Read the model definition and answer for the solid it produces. Units are mm, in the model's axes. Round coordinates to 2 decimals unless told otherwise and drop trailing zeros. Order: outer loops, then holes, each group sorted by start corner. A loop starts at its lowest first (then second) coordinate and runs counter-clockwise, first axis right, second up. Notation, with made-up numbers: (14.5, 49) - (38.5, 49) arc R34 cw to (38.5, 86) - close; hole circle Ø4 at (2.5, -34). An arc over 180 degrees is marked (long way). Put each result on its own line as item: value. Start each with the question number.
Q1. Section A-A on z = 12.5 is taken. Give the vertices of the cut face in (x, y), then the cut area to 3 significant figures.
Q2. Find the intervals of material crossed by line 1 along Y through (x, z) = (-0.25, 10); line 2 along Z through (x, y) = (0, 11.5); line 3 along X through (y, z) = (-4.25, 7.5), in increasing order. Write a range as from..to.
Q3. Section C-C on y = -2 is taken. Give the vertices of the cut face in (x, z), then the cut area to 3 significant figures.
Q4. This flat-tipped pin is pushed along its axis until it touches: pin 1 Ø0.6 at (x, y) = (-4, 7.5) entering from +Z. Where does it stop, or does it pass through?
Q5. Section B-B on y = 10.5 is taken. Give the vertices of the cut face in (x, z).
Q6. Section D-D on z = 3.5 is taken. Give the vertices of the cut face in (x, y), then the cut area to 3 significant figures.
from build123d import *

# Parameters (mm, degrees)
SKETCH027_W     = 15
SKETCH027_H     = 30
PAD008_DEPTH    = 15
SKETCH028_R     = 2
POCKET019_DEPTH = 29
SKETCH029_W     = 0.5
SKETCH029_H     = 17
POCKET020_DEPTH = 10
SKETCH030_W     = 7.783355
SKETCH030_H     = 0.5
POCKET021_DEPTH = 12
FILLET010_R     = 1.5
CHAMFER005_SIZE = 1


with BuildPart() as part:
    # Sketch027 → Pad008 (new body)
    with BuildSketch(Plane.XY):
        Rectangle(SKETCH027_W, SKETCH027_H)
    extrude(amount=PAD008_DEPTH)

    # Sketch028 (on Face3 of Pad008) → Pocket019 (cut)
    with BuildSketch(Plane.XZ.offset(15)):
        with Locations((0, 7.5)):
            Circle(SKETCH028_R)
    extrude(amount=-POCKET019_DEPTH, mode=Mode.SUBTRACT)

    # Sketch029 (on Face5 of Pocket019) → Pocket020 (cut)
    with BuildSketch(Plane.XY.offset(15)):
        with Locations((0.25, 0)):
            Rectangle(SKETCH029_W, SKETCH029_H)
    extrude(amount=-POCKET020_DEPTH, mode=Mode.SUBTRACT)

    # Sketch030 (on Face5 of Pocket020) → Pocket021 (cut)
    with BuildSketch(Plane.XY.offset(15)):
        Polygon((0.095277, -7.753875), (-7.818323, -11.679128), (-7.818323, -11.122255), (0.095277, -7.197002), align=None)
        with Locations((-3.7964, 7.45)):
            Rectangle(SKETCH030_W, SKETCH030_H)
    extrude(amount=-POCKET021_DEPTH, mode=Mode.SUBTRACT)

    # Fillet010
    fillet010_edges = [part.edges().sort_by_distance(p)[0] for p in [
        (0, -15, 0),
        (-7.5, 0, 0),
        (7.5, 0, 0),
        (0, 15, 0),
        (7.5, 15, 7.5),
        (-7.5, 15, 7.5),
        (0, 15, 15),
        (7.5, 0, 15),
        (7.5, -15, 7.5),
        (0, -15, 15),
        (-7.5, -15, 7.5),
    ]]
    fillet(fillet010_edges, radius=FILLET010_R)

    # Chamfer005
    chamfer005_edges = [part.edges().sort_by_distance(p)[0] for p in [
        (-2, -15, 7.5),
    ]]
    chamfer(chamfer005_edges, length=CHAMFER005_SIZE)


solid = part.part
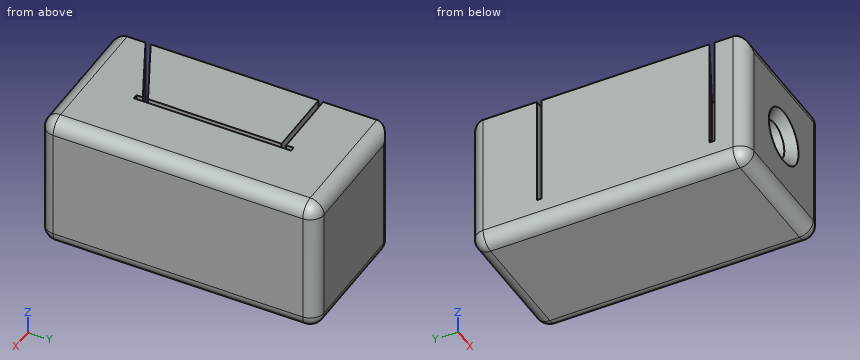
Findings:
1. outline: (-7.5, -13.5) arc R1.5 ccw to (-6, -15) - (6, -15) arc R1.5 ccw to (7.5, -13.5) - (7.5, 13.5) arc R1.5 ccw to (6, 15) - (-6, 15) arc R1.5 ccw to (-7.5, 13.5) - (-7.5, 7.7) - (0, 7.7) - (0, 8.5) - (0.5, 8.5) - (0.5, -8.5) - (0, -8.5) - (0, -7.8) - (-7.5, -11.52) - close; (-7.5, -10.96) - (0, -7.24) - (0, 7.2) - (-7.5, 7.2) - close
1. area: 432 mm2
2. line 1: -14.51..-7.93, -7.37..7.2, 7.7..15
2. line 2: 0..5.5, 9.5..15
2. line 3: -7.5..-2, 2..7.5
3. outline: (-7.5, 1.5) arc R1.5 ccw to (-6, 0) - (6, 0) arc R1.5 ccw to (7.5, 1.5) - (7.5, 13.5) arc R1.5 ccw to (6, 15) - (0.5, 15) - (0.5, 9.44) arc R2 cw to (0.5, 5.56) - (0.5, 5) - (0, 5) - (0, 5.5) arc R2 cw to (0, 9.5) - (0, 15) - (-7.5, 15) - close
3. area: 208 mm2
4. pin 1: z = 15
5. outline: (-7.5, 1.5) arc R1.5 ccw to (-6, 0) - (6, 0) arc R1.5 ccw to (7.5, 1.5) - (7.5, 13.5) arc R1.5 ccw to (6, 15) - (-7.5, 15) - close; hole circle Ø4 at (0, 7.5)
6. outline: (-7.5, -13.5) arc R1.5 ccw to (-6, -15) - (6, -15) arc R1.5 ccw to (7.5, -13.5) - (7.5, 13.5) arc R1.5 ccw to (6, 15) - (-6, 15) arc R1.5 ccw to (-7.5, 13.5) - (-7.5, 7.7) - (0.1, 7.7) - (0.1, 7.2) - (-7.5, 7.2) - (-7.5, -10.96) - (0.1, -7.2) - (0.1, -7.75) - (-7.5, -11.52) - close
6. area: 440 mm2
